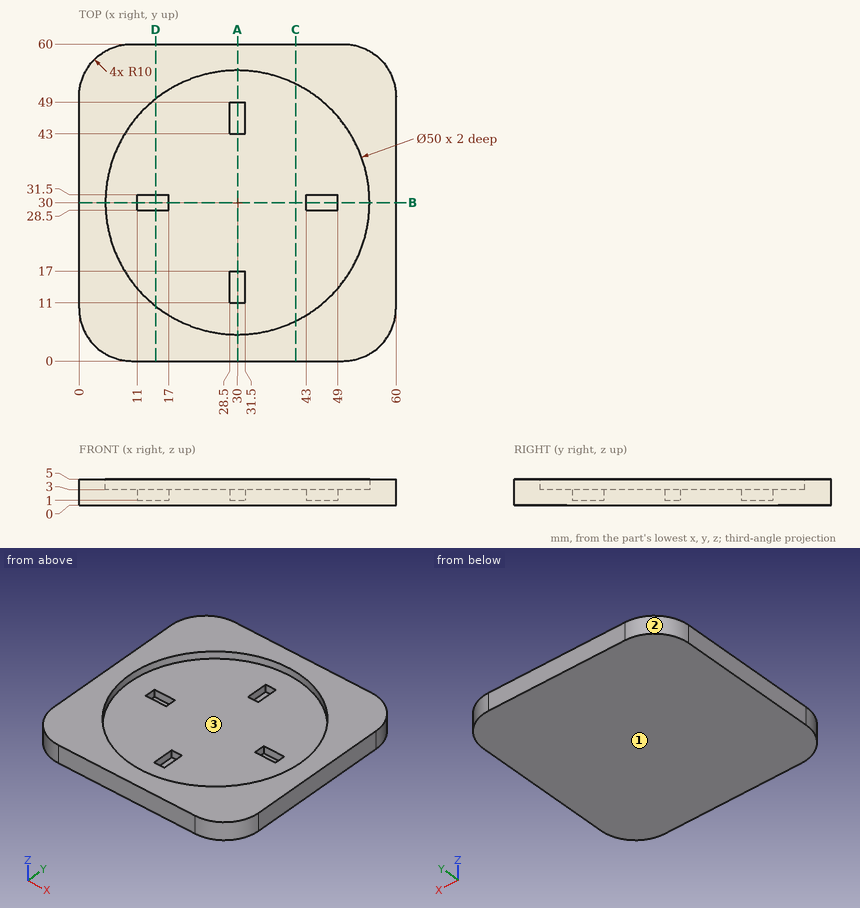
Check sheet for the drawn part. Datum: minimum x, y, z corner. Units: mm. Coordinates: 2 decimals unless noted, no trailing zeros. Order: outer loops, then holes, each group sorted by start corner. A loop starts at its lowest first (then second) coordinate and runs counter-clockwise, first axis right, second up. Notation, with made-up numbers: M 65.25,48 L 71.25,48 A31 ccw 71.25,86 Z; hole C 47,79 d5. An arc over 180 degrees is marked long. One line per question, with ' | ' between items. Start each with the question number.
Item 1: Gauge pin test, flat ends, axial feed: P1, Ø2, axis at y = 30, z = 2, coming from the -X side; P2, Ø2.5, axis at x = 46, y = 29.5, coming from the +Z side; P3, Ø1.5, axis at x = 13, y = 29.5, coming from the +Z side. Record the tip position at first contact, or that the pin passes through.
Item 2: Sectioned sample at C-C on x = 41. Record the cut outline in (y, z).
Item 3: Material ranges on line 1 (Y direction, x = 30.5, z = 2.9); line 2 (Y direction, x = 30, z = 3.55); line 3 (Y direction, x = 45, z = 4.15), recorded low to high.
Item 4: Mould release check, pull along Y, two halves, no side actions. Record for the marked faces 1, 2 and 3: pulls with the +Y half, pulls with the -Y half, needs draft (parallel to the pull), parting line crosses it, or undercut.
Item 5: Sectioned sample at D-D on x = 14.5. Record the cut outline in (y, z), and give its area (3 significant figures).
Item 6: Sectioned sample at A-A on x = 30. Record the cut outline in (y, z), and give its area (3 significant figures).
Answer below:
1) P1: stops at x = 0 | P2: stops at z = 3 | P3: stops at z = 1
2) outline: M 0,0 L 60,0 L 60,5 L 52.45,5 L 52.45,3 L 7.55,3 L 7.55,5 L 0,5 Z
3) line 1: y = 0 to 11, 17 to 43, 49 to 60 | line 2: y = 0 to 5, 55 to 60 | line 3: y = 0 to 10, 50 to 60
4) face 1: needs draft | face 2: pulls with the +Y half | face 3: undercut
5) outline: M 0,0 L 60,0 L 60,5 L 49.62,5 L 49.62,3 L 31.5,3 L 31.5,1 L 28.5,1 L 28.5,3 L 10.38,3 L 10.38,5 L 0,5 Z | area: 216 mm^2
6) outline: M 0,0 L 60,0 L 60,5 L 55,5 L 55,3 L 49,3 L 49,1 L 43,1 L 43,3 L 17,3 L 17,1 L 11,1 L 11,3 L 5,3 L 5,5 L 0,5 Z | area: 176 mm^2
